from build123d import *

# Parameters (mm, degrees)
F0_W     = 120.65
F0_H     = 38.1
F1_DEPTH = 79.375
F2_R     = 31.0007
F3_DEPTH = 38.101
F4_R     = 31.0007
F4_R_2   = 27.8257
F5_DEPTH = 6.35
F6_R     = 8.334375
F7_DEPTH = 79.376


with BuildPart() as f1:
    # F0 (on Front) → F1 (new body)
    with BuildSketch(Plane.XZ):
        with Locations((60.325, 19.05)):
            Rectangle(F0_W, F0_H)
    extrude(amount=F1_DEPTH)

    # F2 (on face) → F3 (cut, through all)
    with BuildSketch(Plane.XY.offset(38.1)):
        with Locations((60.325, -39.6875)):
            Circle(F2_R)
    extrude(amount=-F3_DEPTH, mode=Mode.SUBTRACT)

    # F4 (on face) → F5 (join)
    with BuildSketch(Plane(origin=(0, 0, 0), x_dir=(1, 0, 0), z_dir=(0, 0, -1))):
        with Locations((60.325, 39.6875)):
            Circle(F4_R)
        with Locations((60.325, 39.6875)):
            Circle(F4_R_2, mode=Mode.SUBTRACT)
    extrude(amount=-F5_DEPTH)

    # F6 (on face) → F7 (cut, through all)
    with BuildSketch(Plane.XZ.offset(79.375)):
        with Locations((15.875, 19.05)):
            Circle(F6_R)
        with Locations((104.775, 19.05)):
            Circle(F6_R)
    extrude(amount=-F7_DEPTH, mode=Mode.SUBTRACT)


solid = f1.part
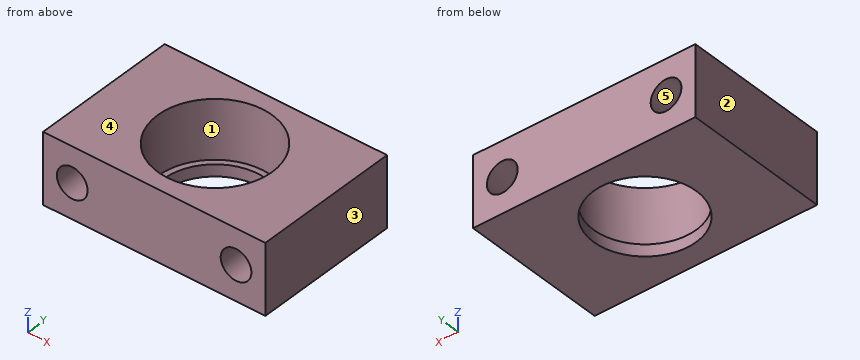
The listing builds one solid part. Answer for the finished solid, in the listing's coordinates (mm). Face numbers are marked on the shaded views. A direction names the side the tool comes from. Coordinates: 2 decimals unless noted, no trailing zeros. Loops run counter-clockwise (first coordinate to the right, second up) from the corner with the lowest first, then second, coordinate; pieces in that order, holes last. Notation, with made-up numbers: (17.25, -16) -> (45.25, -16) arc R15 ccw to (45.25, -11) -> close; hole circle Ø9 at (13, -1.75). An arc over 180 degrees is marked (long way). Write item = value, one per line. Start each with the question number.
1) Straight lines are drawn through the part: line 1 (X direction, y = -15, z = 20); line 2 (X direction, y = -26, z = 29); line 3 (X direction, y = -39, z = 26). For each, find the intervals that lie inside material, in ascending order. Write a range as from..to.
2) A tool of negligible diameter and unlimited length cuts with its end or side. For the marked faces 1 and 2, from which of +Z, -Z, +X, -X, +Y, -Y can it reach the whole face along a straight path? Write none if from no direction.
3) A cutting plane is placed at A-A (z = 19.05). Count the separate pieces of the cut face and the enclosed holes in it, then the cut area to 3 significant figures.
4) Given pin 1 Ø10 at (y, z) = (-44.5, 33) entering from -X, flat-ended and moving along its own axis, determine where the tip first touches the part or whether it passes through.
5) The mould has two halves that part along Z. Classify the marked faces 3, 4 and 5: released by +Z, released by -Z, zero draft, split by the parting line, or undercut.
6) A cutting plane is placed at B-B (y = -52). Give the vertices of the cut face in (x, z) (3 decimals).
7) A cutting plane is placed at D-D (y = -42). Give the vertices of the cut face in (x, z) (3 decimals), then the cut area to 3 significant figures.
8) A cutting plane is placed at C-C (x = 99.5). Give the vertices of the cut face in (y, z) (3 decimals), then the cut area to 3 significant figures.
Responses:
q1.line_1 = 0..7.59, 24.16..41.57, 79.08..96.49, 113.06..120.65
q1.line_2 = 0..32.51, 88.14..120.65
q1.line_3 = 0..11.28, 20.47..29.33, 91.32..100.18, 109.37..120.65
q2.face_1 = +Z
q2.face_2 = +Z, -Z, -X, +Y, -Y
q3.separate_pieces = 3
q3.enclosed_holes = 1
q3.area = 3,910 mm²
q4.pin_1 = 0
q5.face_3 = zero draft
q5.face_4 = released by +Z
q5.face_5 = undercut
q6.outline = (0, 0) -> (35.372, 0) -> (35.372, 6.35) -> (31.874, 6.35) -> (31.874, 38.1) -> (0, 38.1) -> close; (85.278, 0) -> (120.65, 0) -> (120.65, 38.1) -> (88.776, 38.1) -> (88.776, 6.35) -> (85.278, 6.35) -> close; hole circle Ø16.669 at (15.875, 19.05); hole circle Ø16.669 at (104.775, 19.05)
q7.outline = (0, 0) -> (32.596, 0) -> (32.596, 6.35) -> (29.411, 6.35) -> (29.411, 38.1) -> (0, 38.1) -> close; (88.054, 0) -> (120.65, 0) -> (120.65, 38.1) -> (91.239, 38.1) -> (91.239, 6.35) -> (88.054, 6.35) -> close; hole circle Ø16.669 at (15.875, 19.05); hole circle Ø16.669 at (104.775, 19.05)
q7.area = 1,850 mm²
q8.outline = (-79.375, 0) -> (0, 0) -> (0, 12.597) -> (-79.375, 12.597) -> close; (-79.375, 25.503) -> (0, 25.503) -> (0, 38.1) -> (-79.375, 38.1) -> close
q8.area = 2,000 mm²
